Build history of the part. All positions in model axes, mm. Round coordinates to 2 decimals unless told otherwise and drop trailing zeros. Write each loop counter-clockwise with the first axis right and the second up, starting at its lowest first coordinate (ties: lowest second). Pieces come first, ordered by that corner, then holes.
1) Flat gauge pins, fed straight in: pin 1 (6 mm diameter, centred on x = 4, y = 14.5, fed in from -Z); pin 2 (1 mm diameter, centred on y = 3, z = 1.5, fed in from -X); pin 3 (6 mm diameter, centred on x = 2, y = 8.5, fed in from +Z). Where does each tip first touch, or does it go through?
2) Pull direction Y, two halves, no side cores. Call faces 1 (the cylindrical face through (0.54, 7.4, 2.44)), 2 (the flat face through (0, -2, 0)), 3 (the flat face through (0, 17, 0)): +Y half, -Y half, draft (parallel to the pull), parting line (faces both ways), or undercut.
3) Wall check: probe 1 along Y at (x, z) = (-0.25, -3); probe 2 along Y at (x, z) = (-2.5, 3.5); probe 3 along Z at (x, y) = (-1.5, 13.5). Give the ranges that are in metal, low to high.
4) Saw through at D-D (y = 16). Write the cut outline in (x, z), plus the area to 3 significant figures.
5) Saw through at C-C (y = 10.25). Write the cut outline in (x, z), plus the area to 3 significant figures.
Autodesk Inventor part; units mm, degrees
ref_plane "YZ Plane" through (0, 0, 0) normal (1, 0, 0) x (0, 1, 0)
ref_plane "XZ Plane" through (0, 0, 0) normal (0, 1, 0) x (-1, 0, 0)
ref_plane "XY Plane" through (0, 0, 0) normal (0, 0, 1) x (1, 0, 0)
sketch "Szkic1" plane through (0, 0, 0) normal (0, 1, 0) x (-1, 0, 0)
  circle A0 centre (0, 0) radius 2.5
  circle A1 centre (0, 0) radius 5
  dimension "d0" = 5
  dimension "d1" = 10
extrude "Wyciągnięcie proste1" add sketch "Szkic1" against normal blind 2 contours A0 | A1
extrude "Wyciągnięcie proste2" add sketch "Szkic1" along normal blind 17 contours A0 | A1
extrude "Wyciągnięcie proste3" cut sketch "Szkic1" along normal blind 15
fillet "Zaokrąglenie1" radius 2 2 edges at (5, 17, 0) (5, -2, 0)
properties part number "nit_skrecany" material "Aluminium"
Evaluation:
1. pin 1: stops at z = -4.89
1. pin 2: stops at x = -2.29
1. pin 3: stops at z = 2.5
2. face 1: undercut
2. face 2: -Y half
2. face 3: +Y half
3. probe 1: y = -2 to 0, 15 to 17
3. probe 2: y = -1.52 to 0, 15 to 16.52
3. probe 3: z = -2 to 2
4. outline: circle Ø9.46 at (0, 0)
4. area: 70.4 mm2
5. outline: circle Ø5 at (0, 0)
5. area: 19.6 mm2
